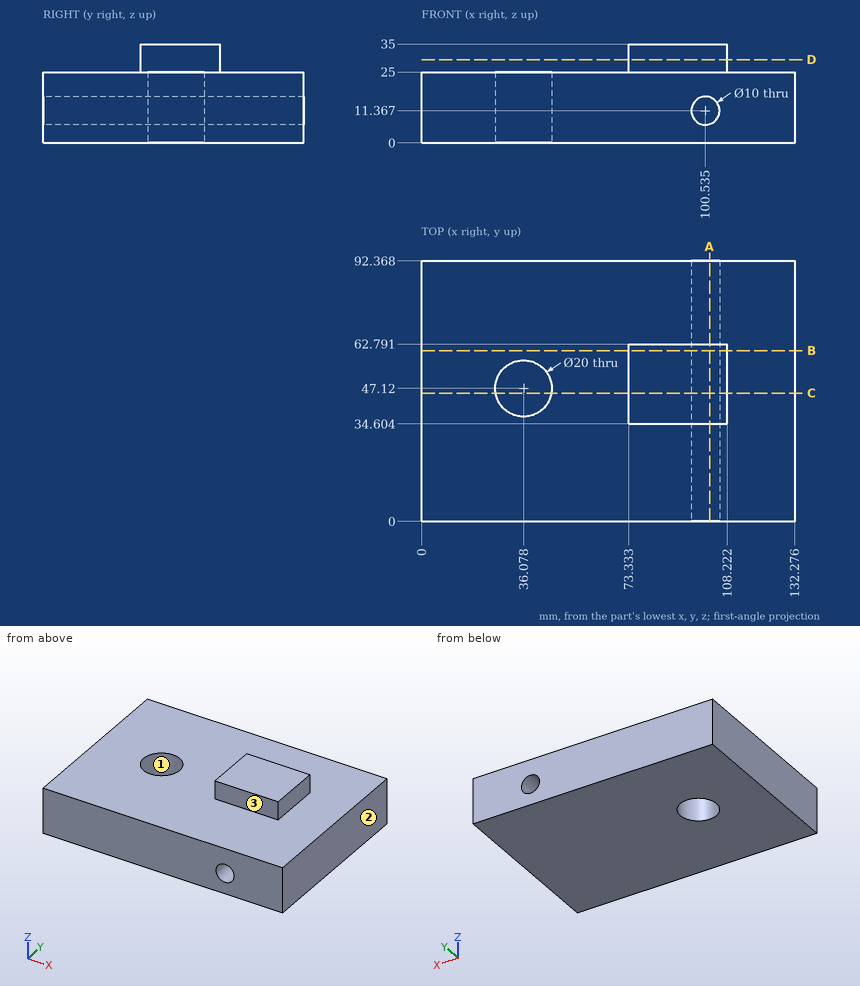
Source: three-view drawing plus pictorial views. Frame: mm from the lowest corner of the part. Round coordinates to 2 decimals unless told otherwise and drop trailing zeros. Loops run counter-clockwise (first coordinate to the right, second up) from the corner with the lowest first, then second, coordinate; pieces in that order, holes last. Notation, with made-up numbers: M 52.5,50 L 88.5,50 A33 cw 88.5,82 Z; hole C 24.25,16.25 d8. An arc over 180 degrees is marked long. Put each result on its own line as item: value.
(1) Pull-direction query (Y, two-part tool) for the marked faces 1, 2 and 3; classes: released by +Y, released by -Y, zero draft, split by the parting line, or undercut.
Solutions:
face 1: undercut
face 2: zero draft
face 3: released by -Y
(2) First-contact query: pin 1 (12 mm diameter, centred on x = 105.5, y = 71.5, fed in from +Z); pin 2 (5 mm diameter, centred on y = 50, z = 29, fed in from -X); pin 3 (3 mm diameter, centred on x = 97.5, z = 29, fed in from +Y); pin 4 (9 mm diameter, centred on x = 100.53, z = 11.37, fed in from -Y). Flat tips, straight axial feed; report the tip coordinate or a pass-through.
Solutions:
pin 1: z = 25
pin 2: x = 73.33
pin 3: y = 62.79
pin 4: through
(3) Section C-C, the plane y = 45.5. Return loops of the section in (x, z) (1 decimal).
Solutions:
outline: M 0,0 L 26.2,0 L 26.2,25 L 0,25 Z; M 45.9,0 L 132.3,0 L 132.3,25 L 108.2,25 L 108.2,35 L 73.3,35 L 73.3,25 L 45.9,25 Z; hole C 100.5,11.4 d10
(4) Section B-B, the plane y = 60.5. Return loops of the section in (x, z) (1 decimal), and give its area (3 significant figures).
Solutions:
outline: M 0,0 L 132.3,0 L 132.3,25 L 108.2,25 L 108.2,35 L 73.3,35 L 73.3,25 L 0,25 Z; hole C 100.5,11.4 d10
area: 3,580 mm²
(5) Section D-D, the plane z = 29.5. Return loops of the section in (x, y).
Solutions:
outline: M 73.33,34.6 L 108.22,34.6 L 108.22,62.79 L 73.33,62.79 Z
(6) Ray query, line 1 (X direction, y = 59.5, z = 11) (1 decimal); line 2 (Z direction, x = 93, y = 64); line 3 (X direction, y = 66.5, z = 15) (1 decimal). Return the intervals inside material, ascending. Write a range as [from, to].
Solutions:
line 1: [0, 95.5], [105.5, 132.3]
line 2: [0, 25]
line 3: [0, 97.1], [104, 132.3]
(7) Section A-A, the plane x = 102. Return loops of the section in (y, z), and give its area (3 significant figures).
Solutions:
outline: M 0,0 L 92.37,0 L 92.37,6.59 L 0,6.59 Z; M 0,16.15 L 92.37,16.15 L 92.37,25 L 62.79,25 L 62.79,35 L 34.6,35 L 34.6,25 L 0,25 Z
area: 1,710 mm²
